Drawing for the job (mm, zero at the part's lowest x, y, z). A direction names the side the tool comes from. Coordinates: 2 decimals unless noted, no trailing zeros. Write each loop counter-clockwise with the first axis right and the second up, starting at its lowest first coordinate (ties: lowest second). Pieces come first, ordered by that corner, then holes. Notation, with made-up numbers: (2.25, -27.5) -> (40.25, -27.5) arc R9 ccw to (40.25, -10.5) -> close; hole circle Ø1 at (73.25, 71). An arc over 180 degrees is marked (long way). Write item = value, one per line. Start each with the question number.
Q1. Pin check, flat tips, straight feed: P1, Ø2, axis at x = 37, y = 28, coming from the -Z side; P2, Ø3.5, axis at x = 5, z = 11, coming from the +Y side; P3, Ø1.5, axis at x = 13, y = 44, coming from the +Z side; P4, Ø1.5, axis at y = 44, z = 4.5, coming from the -X side. Stop position of each tip, or through.
Q2. Probe line 1 (Z direction, x = 11.25, y = 23.5); line 2 (Z direction, x = 8, y = 45); line 3 (Y direction, x = 42.5, z = 5.5). List the from-to ranges inside material, lowest first.
Q3. Tool access for the marked faces 1, 2 and 3: list every direction of +Z, -Z, +X, -X, +Y, -Y with a clear straight run to the whole face (end or side of a thin tool).
Q4. Band-saw the part on C-C, the plane z = 12.25. List the corners of the cut face in (x, y), plus the area to 3 significant figures.
Q5. Band-saw the part on B-B, the plane x = 11.25. List the corners of the cut face in (y, z), plus the area to 3 significant figures.
Q6. Band-saw the part on A-A, the plane z = 8. List the corners of the cut face in (x, y), plus the area to 3 significant figures.
Q7. Band-saw the part on D-D, the plane x = 45. List the corners of the cut face in (y, z).
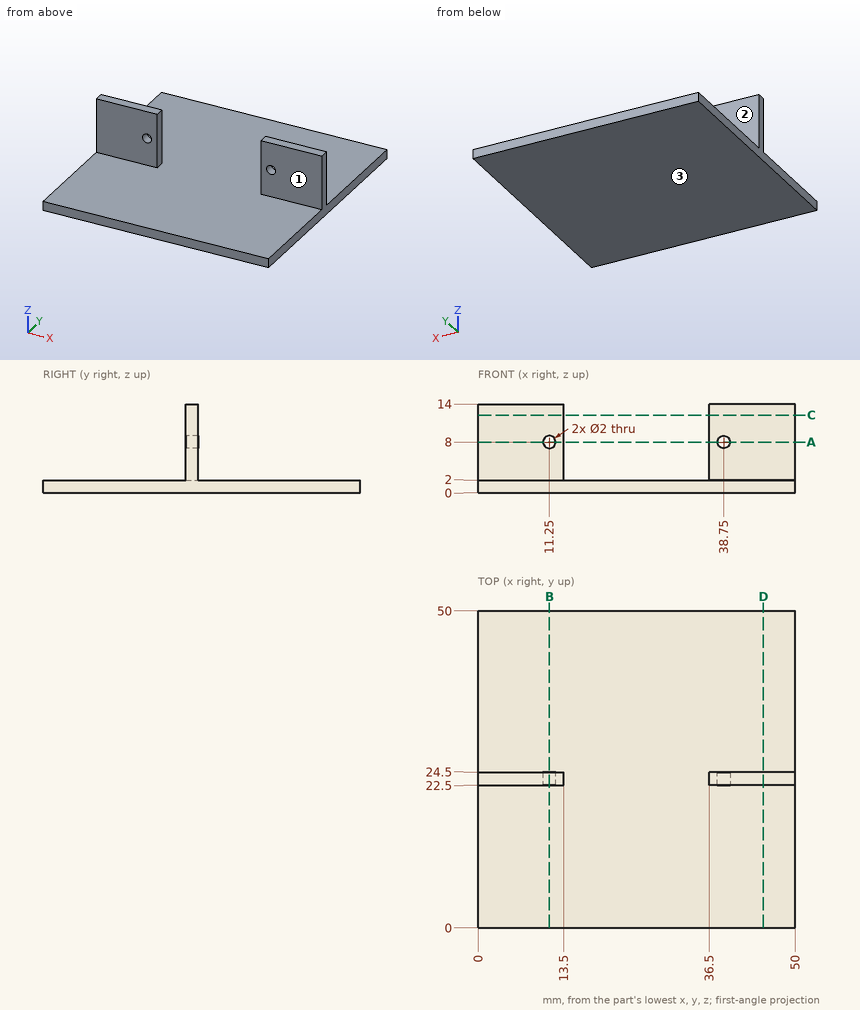
Ans:
q1.P1 = 0
q1.P2 = 24.5
q1.P3 = 2
q1.P4 = through
q2.line_1 = 0 to 7, 9 to 14
q2.line_2 = 0 to 2
q2.line_3 = 22.5 to 24.5
q3.face_1 = +Z, +X, -X, -Y
q3.face_2 = +Z, +X, -X, +Y
q3.face_3 = -Z, +X, -X, +Y, -Y
q4.outline = (0, 22.5) -> (13.5, 22.5) -> (13.5, 24.5) -> (0, 24.5) -> close; (36.5, 22.5) -> (50, 22.5) -> (50, 24.5) -> (36.5, 24.5) -> close
q4.area = 54.0 mm2
q5.outline = (0, 0) -> (50, 0) -> (50, 2) -> (24.5, 2) -> (24.5, 7) -> (22.5, 7) -> (22.5, 2) -> (0, 2) -> close; (22.5, 9) -> (24.5, 9) -> (24.5, 14) -> (22.5, 14) -> close
q5.area = 120 mm2
q6.outline = (0, 22.5) -> (10.25, 22.5) -> (10.25, 24.5) -> (0, 24.5) -> close; (12.25, 22.5) -> (13.5, 22.5) -> (13.5, 24.5) -> (12.25, 24.5) -> close; (36.5, 22.5) -> (37.75, 22.5) -> (37.75, 24.5) -> (36.5, 24.5) -> close; (39.75, 22.5) -> (50, 22.5) -> (50, 24.5) -> (39.75, 24.5) -> close
q6.area = 46.0 mm2
q7.outline = (0, 0) -> (50, 0) -> (50, 2) -> (24.5, 2) -> (24.5, 14) -> (22.5, 14) -> (22.5, 2) -> (0, 2) -> close
